```python
from build123d import *

# Parameters (mm, degrees)
F0_W          = 154
F0_H          = 74
F1_DEPTH      = 30
F2_R          = 10
F3_DEPTH      = 180
F3_DEPTH_BACK = 25


with BuildPart() as f1:
    # F0 (on Top) → F1 (new body)
    with BuildSketch(Plane.XY):
        Rectangle(F0_W, F0_H)
    extrude(amount=F1_DEPTH)

    # F2 (on face) → F3 (join, two sides)
    with BuildSketch(Plane.YZ.offset(77)) as f3_sk:
        with Locations((0, 15)):
            Circle(F2_R)
    extrude(amount=-F3_DEPTH)
    extrude(f3_sk.sketch, amount=F3_DEPTH_BACK)


solid = f1.part
```
Source: CAD feature listing. Evaluate the final solid. Frame: model axes, mm. A direction names the side the tool comes from. Coordinates: 2 decimals unless noted, no trailing zeros. Loops run counter-clockwise (first coordinate to the right, second up) from the corner with the lowest first, then second, coordinate; pieces in that order, holes last. Notation, with made-up numbers: (50.25, 46) - (99.25, 46) arc R15 cw to (99.25, 63) - close; hole circle Ø6 at (6.5, -20.75). An arc over 180 degrees is marked (long way). Answer as CSV lines item,"result".
1. Section C-C (x = -84). Return loops of the section in (y, z), then the cut area to 3 significant figures.
Established:
outline,"circle Ø20 at (0, 15)"
area,"314 mm2"
2. Ray query, line 1 (X direction, y = -10.5, z = 2); line 2 (Y direction, x = 78.5, z = 24.25); line 3 (Z direction, x = -77.5, y = -2.5). Return the intervals inside material, ascending.
Established:
line 1,"x = -77 to 77"
line 2,"y = -3.8 to 3.8"
line 3,"z = 5.32 to 24.68"
3. Section A-A (y = 0). Return loops of the section in (x, z).
Established:
outline,"(-103, 5) - (-77, 5) - (-77, 0) - (77, 0) - (77, 5) - (102, 5) - (102, 25) - (77, 25) - (77, 30) - (-77, 30) - (-77, 25) - (-103, 25) - close"
4. Reachability of faces 1 (the flat face through (-103, 0, 15)), 2 (the cylindrical face through (89.325, -1.302, 24.915)), 3 (the cylindrical face through (-89.818, -1.302, 24.915)) from +Z, -Z, +X, -X, +Y, -Y: full face, straight path, thin tool, end or side. Return the list, or none.
Established:
face 1,"+Z, -Z, -X, +Y, -Y"
face 2,"+X"
face 3,"-X"
5. Contact query for flat-ended pins moving along their axis: pin 1 (4 mm diameter, centred on y = -14, z = 21, fed in from -X); pin 2 (10 mm diameter, centred on y = 17, z = 9, fed in from +X); pin 3 (3 mm diameter, centred on x = 80, z = 24.5, fed in from -Y). Output: stop coordinate, or through.
Established:
pin 1,"stops at x = -77"
pin 2,"stops at x = 77"
pin 3,"stops at y = -6"
6. Section D-D (y = -16.5). Return loops of the section in (x, z).
Established:
outline,"(-77, 0) - (77, 0) - (77, 30) - (-77, 30) - close"
7. Section B-B (z = 15). Return loops of the section in (x, y), then the cut area to 3 significant figures.
Established:
outline,"(-103, -10) - (-77, -10) - (-77, -37) - (77, -37) - (77, -10) - (102, -10) - (102, 10) - (77, 10) - (77, 37) - (-77, 37) - (-77, 10) - (-103, 10) - close"
area,"12,400 mm2"
